Verification items for the finished model (mm, model axes). Face numbers are marked on the shaded views. A direction names the side the tool comes from. Give positions to 0.01 mm unless a question says otherwise; leave off trailing zeros. Write each loop counter-clockwise with the first axis right and the second up, starting at its lowest first coordinate (ties: lowest second). Pieces come first, ordered by that corner, then holes. Notation, with made-up numbers: (56, 66.25) -> (67, 66.25) arc R20 cw to (67, 81.25) -> close; hole circle Ø3 at (-2.75, -29.75). An arc over 180 degrees is marked (long way). Write item = value, one per line.
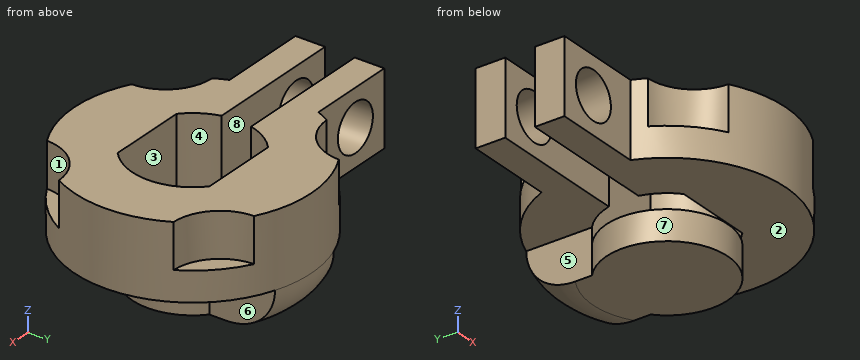
from build123d import *

# Parameters (mm, degrees)
SKETCH_1_R          = 14
SKETCH_1_R_2        = 1.5
EXTRUDE_1_DEPTH     = 2
CUT_EXTRUDE_1_DEPTH = 20.899748742
EXTRUDE_4_DEPTH     = 2.5
EXTRUDE_START       = 5
SKETCH_6_R          = 8
EXTRUDE_5_DEPTH     = 5
EXTRUDE_START_2     = 1
EXTRUDE_6_DEPTH     = 1
SKETCH_8_W          = 8
SKETCH_8_H          = 2
EXTRUDE_7_DEPTH     = 5
SKETCH_9_R          = 1.6
CUT_EXTRUDE_3_DEPTH = 24.606143268
EXTRUDE_START_3     = 2
EXTRUDE_8_DEPTH     = 2
SKETCH_11_W         = 12.041493288
SKETCH_11_H         = 2
CUT_EXTRUDE_4_DEPTH = 5
FILLET_2_R          = 3
CUT_EXTRUDE_START   = -4.5
SKETCH_12_R         = 14
CUT_EXTRUDE_5_DEPTH = 4.5
SKETCH_13_R         = 3.2
CUT_EXTRUDE_6_DEPTH = 3


with BuildPart() as part:
    # Sketch 1 → Extrude 1 (new body)
    with BuildSketch(Plane.XY):
        Circle(SKETCH_1_R)
        with Locations((-7.071067812, 7.071067812)):
            Circle(SKETCH_1_R_2, mode=Mode.SUBTRACT)
        with Locations((7.071067812, 7.071067812)):
            Circle(SKETCH_1_R_2, mode=Mode.SUBTRACT)
        with Locations((-7.071067812, -7.071067812)):
            Circle(SKETCH_1_R_2, mode=Mode.SUBTRACT)
        with Locations((7.071067812, -7.071067812)):
            Circle(SKETCH_1_R_2, mode=Mode.SUBTRACT)
    extrude(amount=EXTRUDE_1_DEPTH)

    # Sketch 2 → Cut-Extrude 1 (cut, through all)
    with BuildSketch(Plane(origin=(0, 0, 0), x_dir=(-1, 0, 0), z_dir=(0, 0, -1))):
        with BuildLine():
            ThreePointArc((-2.683281573, 3.1), (-4.1, 0), (-2.683281573, -3.1))
            Line((-2.683281573, -3.1), (2.683281573, -3.1))
            ThreePointArc((2.683281573, -3.1), (4.1, 0), (2.683281573, 3.1))
            Line((2.683281573, 3.1), (-2.683281573, 3.1))
        make_face()
    extrude(amount=-CUT_EXTRUDE_1_DEPTH, mode=Mode.SUBTRACT)

    # Sketch 3 → Extrude 4 (add)
    with BuildSketch(Plane(origin=(0, 0, 0), x_dir=(-1, 0, 0), z_dir=(0, 0, -1))):
        Polygon((0, 3.1), (3.7, 3.1), (3.7, 7.1), (-3.7, 7.1), (-3.7, 3.1), align=None)
    extrude(amount=EXTRUDE_4_DEPTH)

    # Sketch 6 → Extrude 5 (add)
    with BuildSketch(Plane(origin=(0, 0, -2.5), x_dir=(-1, 0, 0), z_dir=(0, 0, -1)).offset(EXTRUDE_START)):
        with Locations(Location((0, 0, 0), (0, 0, 117.548545959))):
            Circle(SKETCH_6_R)
        with BuildLine():
            Line((-2.683281573, -3.1), (2.683281573, -3.1))
            ThreePointArc((2.683281573, -3.1), (4.1, 0), (2.683281573, 3.1))
            Line((2.683281573, 3.1), (-2.683281573, 3.1))
            ThreePointArc((-2.683281573, 3.1), (-4.1, 0), (-2.683281573, -3.1))
        make_face(mode=Mode.SUBTRACT)
    extrude(amount=-EXTRUDE_5_DEPTH)

    # Sketch 7 → Extrude 6 (add)
    with BuildSketch(Plane(origin=(0, 0, -7.5), x_dir=(-1, 0, 0), z_dir=(0, 0, -1)).offset(EXTRUDE_START_2)):
        with BuildLine():
            Line((-2.683281573, 3.1), (-2.683281573, 7.536577473))
            ThreePointArc((-2.683281573, 7.536577473), (0, 8), (2.683281573, 7.536577473))
            Line((2.683281573, 7.536577473), (2.683281573, 3.1))
            Line((2.683281573, 3.1), (-2.683281573, 3.1))
        make_face()
    extrude(amount=-EXTRUDE_6_DEPTH)

    # Sketch 8 → Extrude 7 (add)
    with BuildSketch(Plane(origin=(0, 0, -7.5), x_dir=(-1, 0, 0), z_dir=(0, 0, -1))):
        with Locations((9.447401339, 2)):
            Rectangle(SKETCH_8_W, SKETCH_8_H)
        with Locations((9.447401339, -2)):
            Rectangle(SKETCH_8_W, SKETCH_8_H)
    extrude(amount=-EXTRUDE_7_DEPTH)

    # Sketch 9 → Cut-Extrude 3 (cut, through all)
    with BuildSketch(Plane(origin=(0, 3, 0), x_dir=(1, 0, 0), z_dir=(0, 1, 0))):
        with Locations(Location((-10.8, 5, 0), (0, 0, 180))):
            Circle(SKETCH_9_R)
    extrude(amount=-CUT_EXTRUDE_3_DEPTH, mode=Mode.SUBTRACT)

    # Sketch 10 → Extrude 8 (add)
    with BuildSketch(Plane(origin=(0, 0, -8.5), x_dir=(-1, 0, 0), z_dir=(0, 0, -1)).offset(EXTRUDE_START_3)):
        with BuildLine():
            Line((-2.683281573, 7.536577473), (-2.683281573, 3.1))
            ThreePointArc((-2.683281573, 3.1), (0, -4.1), (2.683281573, 3.1))
            Line((2.683281573, 3.1), (2.683281573, 7.536577473))
            ThreePointArc((2.683281573, 7.536577473), (0, 8), (-2.683281573, 7.536577473))
        make_face()
    extrude(amount=-EXTRUDE_8_DEPTH)

    # Sketch 11 → Cut-Extrude 4 (cut)
    with BuildSketch(Plane(origin=(0, 0, -7.5), x_dir=(-1, 0, 0), z_dir=(0, 0, -1))):
        with Locations((7.426654695, 0)):
            Rectangle(SKETCH_11_W, SKETCH_11_H)
    extrude(amount=-CUT_EXTRUDE_4_DEPTH, mode=Mode.SUBTRACT)

    # Fillet 2
    # the kernel refuses this fillet: 3 mm, written as the material it takes off along each edge
    with BuildSketch(Plane(origin=(0, 0, -10.5), x_dir=(-0.9579045500922062, 0.28708687345932127, 0), z_dir=(-0.28708687345932127, -0.9579045500922062, 0))) as fillet_2_piece_1:
        with BuildLine():
            CenterArc((8 - FILLET_2_R, -FILLET_2_R), FILLET_2_R, 0, 90)
            Line((8 - FILLET_2_R, 0), (8, 0))
            Line((8, 0), (8, -FILLET_2_R))
        make_face()
    revolve(axis=Axis((0, 0, -10.5), (0, 0, -1)), revolution_arc=146.632736988, mode=Mode.SUBTRACT)

    # Sketch 12 → Cut-Extrude 5 (cut)
    with BuildSketch(Plane.XY.offset(2).offset(CUT_EXTRUDE_START)):
        Circle(SKETCH_12_R)
    extrude(amount=CUT_EXTRUDE_5_DEPTH, mode=Mode.SUBTRACT)

    # Sketch 13 → Cut-Extrude 6 (cut)
    with BuildSketch(Plane.XY.offset(-2.5)):
        with Locations((-7.071067812, 7.071067812)):
            Circle(SKETCH_13_R)
        with Locations((7.071067812, 7.071067812)):
            Circle(SKETCH_13_R)
        with Locations((-7.071067812, -7.071067812)):
            Circle(SKETCH_13_R)
        with Locations((7.071067812, -7.071067812)):
            Circle(SKETCH_13_R)
    extrude(amount=-CUT_EXTRUDE_6_DEPTH, mode=Mode.SUBTRACT)


solid = part.part
Item 1: Sectioned sample at B-B on z = -5. Record the cut outline in (x, y).
Response values:
outline = (-13.45, -3) -> (-12.4, -3) -> (-12.4, -1) -> (-13.45, -1) -> close; (-13.45, 1) -> (-12.4, 1) -> (-12.4, 3) -> (-13.45, 3) -> close; (-9.2, -3) -> (-7.42, -3) arc R8 ccw to (-7, -3.87) arc R3.2 cw to (-3.87, -7) arc R8 ccw to (3.87, -7) arc R3.2 cw to (7, -3.87) arc R8 ccw to (7, 3.87) arc R3.2 cw to (3.87, 7) arc R8 ccw to (-3.87, 7) arc R3.2 cw to (-7, 3.87) arc R8 ccw to (-7.42, 3) -> (-9.2, 3) -> (-9.2, 1) -> (-3.98, 1) arc R4.1 cw to (-2.68, 3.1) -> (2.68, 3.1) arc R4.1 cw to (2.68, -3.1) -> (-2.68, -3.1) arc R4.1 cw to (-3.98, -1) -> (-9.2, -1) -> close
Item 2: Go/stop test with flat-tipped pins: P1, Ø1.5, axis at y = 5, z = -9, coming from the +X side; P2, Ø1, axis at y = -4.5, z = -5.5, coming from the -X side; P3, Ø1.5, axis at y = 5.5, z = -9, coming from the -X side; P4, Ø1.9, axis at x = -10.8, z = -5, coming from the +Y side. Record where each tip stops, or that it passes through.
Response values:
P1 = 2.68
P2 = -6.93
P3 = -2.68
P4 = through
Item 3: Sectioned sample at D-D on y = 2.75. Record the cut outline in (x, z), then the cut area to 3 significant figures.
Response values:
outline = (-13.45, -7.5) -> (-3.04, -7.5) -> (-3.04, -2.5) -> (-13.45, -2.5) -> close; (-3.04, -10.5) -> (3.04, -10.5) -> (3.04, -8.5) -> (-3.04, -8.5) -> close; (3.04, -7.5) -> (7.51, -7.5) -> (7.51, -2.5) -> (3.04, -2.5) -> close; hole circle Ø3.2 at (-10.8, -5)
area = 78.5 mm^2
Item 4: Sectioned sample at A-A on y = 0. Record the cut outline in (x, z).
Response values:
outline = (-4.1, -10.5) -> (4.1, -10.5) -> (4.1, -8.5) -> (-4.1, -8.5) -> close; (4.1, -7.5) -> (8, -7.5) -> (8, -2.5) -> (4.1, -2.5) -> close
Item 5: Set-up check for the marked faces 4, 5, 6, 7 and 8: record each of +Z, -Z, +X, -X, +Y, -Y from which the full face is reachable in a straight line by a thin tool's end or side.
Response values:
face_4 = +Z
face_5 = -Z, -X, +Y
face_6 = -Z, +X, +Y
face_7 = -Z
face_8 = +Z, -Z, -X
Item 6: Mould release check, pull along Y, two halves, no side actions. Record for the marked faces 1, 2 and 3: +Y half, -Y half, draft (parallel to the pull), parting line (faces both ways), or undercut.
Response values:
face_1 = -Y half
face_2 = draft
face_3 = undercut
Item 7: Material ranges on line 1 (X direction, y = -2.25, z = -4); line 2 (Z direction, x = -10.8, y = 2); line 3 (X direction, y = -2, z = -4.5), recorded low to high.
Response values:
line_1 = -13.45 to -12.05, -9.55 to -3.43, 3.43 to 7.68
line_2 = -7.5 to -6.6, -3.4 to -2.5
line_3 = -13.45 to -12.32, -9.28 to -3.58, 3.58 to 7.75
Item 8: Sectioned sample at C-C on x = 0. Record the cut outline in (y, z), then the cut area to 3 significant figures.
Response values:
outline = (-8, -7.5) -> (-3.1, -7.5) -> (-3.1, -2.5) -> (-8, -2.5) -> close; (-4.1, -10.5) -> (5, -10.5) arc R3 ccw to (8, -7.5) -> (8, -2.5) -> (3.1, -2.5) -> (3.1, -8.5) -> (-4.1, -8.5) -> close
area = 76.2 mm^2
